from build123d import *

# Parameters (mm, degrees)
SKETCH3_R           = 2.032
SKETCH3_W           = 0.76159928
SKETCH3_H           = 0.76159928
SKETCH3_W_2         = 1.204804675
SKETCH3_H_2         = 2.605195325
SKETCH3_W_3         = 2.605195325
SKETCH3_H_3         = 1.204804675
BOSS_EXTRUDE3_DEPTH = 914.4


with BuildPart() as part:
    # Sketch3 → Boss-Extrude3 (new body)
    with BuildSketch(Plane.XY):
        with BuildLine():
            ThreePointArc((9.717596045, 8.176694142), (8.980256121, 8.980256121), (8.176694142, 9.717596045))
            Line((8.176694142, 9.717596045), (4.57240072, 9.717596045))
            Line((4.57240072, 9.717596045), (4.57240072, 7.11240072))
            Line((4.57240072, 7.11240072), (4.57240072, 5.334))
            Line((4.57240072, 5.334), (5.334, 5.334))
            Line((5.334, 5.334), (5.334, 4.57240072))
            Line((5.334, 4.57240072), (7.11240072, 4.57240072))
            Line((7.11240072, 4.57240072), (9.717596045, 4.57240072))
            Line((9.717596045, 4.57240072), (9.717596045, 8.176694142))
        make_face()
        with Locations((6.914797213, 6.914797213)):
            Circle(SKETCH3_R, mode=Mode.SUBTRACT)
        with Locations((4.95320036, 4.95320036)):
            Rectangle(SKETCH3_W, SKETCH3_H)
        Polygon((4.57240072, 5.334), (3.367596045, 5.334), (3.367596045, 4.191), (4.191, 4.191), (4.191, 3.367596045), (5.334, 3.367596045), (5.334, 4.57240072), (4.57240072, 4.57240072), align=None)
        with BuildLine():
            Line((3.367596045, 5.334), (-3.367596045, 5.334))
            Line((-3.367596045, 5.334), (-3.367596045, 4.191))
            Line((-3.367596045, 4.191), (-2.262062168, 4.191))
            ThreePointArc((-2.262062168, 4.191), (0, 4.7625), (2.262062168, 4.191))
            Line((2.262062168, 4.191), (3.367596045, 4.191))
            Line((3.367596045, 4.191), (3.367596045, 5.334))
        make_face()
        with BuildLine():
            Line((5.334, 3.367596045), (4.191, 3.367596045))
            Line((4.191, 3.367596045), (4.191, 2.262062168))
            ThreePointArc((4.191, 2.262062168), (4.617415064, 1.16656949), (4.7625, 0))
            ThreePointArc((4.7625, 0), (4.617415064, -1.16656949), (4.191, -2.262062168))
            Line((4.191, -2.262062168), (4.191, -3.367596045))
            Line((4.191, -3.367596045), (5.334, -3.367596045))
            Line((5.334, -3.367596045), (5.334, 3.367596045))
        make_face()
        with Locations((3.969998383, 8.414998383)):
            Rectangle(SKETCH3_W_2, SKETCH3_H_2)
        with Locations((8.414998383, 3.969998383)):
            Rectangle(SKETCH3_W_3, SKETCH3_H_3)
        with BuildLine():
            Line((4.57240072, -9.717596045), (8.176694142, -9.717596045))
            ThreePointArc((8.176694142, -9.717596045), (8.980256121, -8.980256121), (9.717596045, -8.176694142))
            Line((9.717596045, -8.176694142), (9.717596045, -4.57240072))
            Line((9.717596045, -4.57240072), (7.11240072, -4.57240072))
            Line((7.11240072, -4.57240072), (5.334, -4.57240072))
            Line((5.334, -4.57240072), (5.334, -5.334))
            Line((5.334, -5.334), (4.57240072, -5.334))
            Line((4.57240072, -5.334), (4.57240072, -7.11240072))
            Line((4.57240072, -7.11240072), (4.57240072, -9.717596045))
        make_face()
        with Locations((6.914797213, -6.914797213)):
            Circle(SKETCH3_R, mode=Mode.SUBTRACT)
        with Locations((4.95320036, -4.95320036)):
            Rectangle(SKETCH3_W, SKETCH3_H)
        with Locations((8.414998383, -3.969998383)):
            Rectangle(SKETCH3_W_3, SKETCH3_H_3)
        with Locations((3.969998383, -8.414998383)):
            Rectangle(SKETCH3_W_2, SKETCH3_H_2)
        Polygon((3.367596045, -4.191), (3.367596045, -5.334), (4.57240072, -5.334), (4.57240072, -4.57240072), (5.334, -4.57240072), (5.334, -3.367596045), (4.191, -3.367596045), (4.191, -4.191), align=None)
        with BuildLine():
            Line((-2.262062168, -4.191), (-3.367596045, -4.191))
            Line((-3.367596045, -4.191), (-3.367596045, -5.334))
            Line((-3.367596045, -5.334), (3.367596045, -5.334))
            Line((3.367596045, -5.334), (3.367596045, -4.191))
            Line((3.367596045, -4.191), (2.262062168, -4.191))
            ThreePointArc((2.262062168, -4.191), (0, -4.7625), (-2.262062168, -4.191))
        make_face()
        with Locations((-4.95320036, -4.95320036)):
            Rectangle(SKETCH3_W, SKETCH3_H)
        Polygon((-4.191, -3.367596045), (-5.334, -3.367596045), (-5.334, -4.57240072), (-4.57240072, -4.57240072), (-4.57240072, -5.334), (-3.367596045, -5.334), (-3.367596045, -4.191), (-4.191, -4.191), align=None)
        with BuildLine():
            Line((-5.334, -4.57240072), (-7.11240072, -4.57240072))
            Line((-7.11240072, -4.57240072), (-9.717596045, -4.57240072))
            Line((-9.717596045, -4.57240072), (-9.717596045, -8.176694142))
            ThreePointArc((-9.717596045, -8.176694142), (-8.980256121, -8.980256121), (-8.176694142, -9.717596045))
            Line((-8.176694142, -9.717596045), (-4.57240072, -9.717596045))
            Line((-4.57240072, -9.717596045), (-4.57240072, -7.11240072))
            Line((-4.57240072, -7.11240072), (-4.57240072, -5.334))
            Line((-4.57240072, -5.334), (-5.334, -5.334))
            Line((-5.334, -5.334), (-5.334, -4.57240072))
        make_face()
        with Locations((-6.914797213, -6.914797213)):
            Circle(SKETCH3_R, mode=Mode.SUBTRACT)
        with Locations((-3.969998383, -8.414998383)):
            Rectangle(SKETCH3_W_2, SKETCH3_H_2)
        with Locations((-8.414998383, -3.969998383)):
            Rectangle(SKETCH3_W_3, SKETCH3_H_3)
        with BuildLine():
            Line((-4.191, 3.367596045), (-5.334, 3.367596045))
            Line((-5.334, 3.367596045), (-5.334, -3.367596045))
            Line((-5.334, -3.367596045), (-4.191, -3.367596045))
            Line((-4.191, -3.367596045), (-4.191, -2.262062168))
            ThreePointArc((-4.191, -2.262062168), (-4.7625, 0), (-4.191, 2.262062168))
            Line((-4.191, 2.262062168), (-4.191, 3.367596045))
        make_face()
        with Locations((-4.95320036, 4.95320036)):
            Rectangle(SKETCH3_W, SKETCH3_H)
        Polygon((-4.57240072, 4.57240072), (-5.334, 4.57240072), (-5.334, 3.367596045), (-4.191, 3.367596045), (-4.191, 4.191), (-3.367596045, 4.191), (-3.367596045, 5.334), (-4.57240072, 5.334), align=None)
        with BuildLine():
            Line((-9.717596045, 4.57240072), (-7.11240072, 4.57240072))
            Line((-7.11240072, 4.57240072), (-5.334, 4.57240072))
            Line((-5.334, 4.57240072), (-5.334, 5.334))
            Line((-5.334, 5.334), (-4.57240072, 5.334))
            Line((-4.57240072, 5.334), (-4.57240072, 7.11240072))
            Line((-4.57240072, 7.11240072), (-4.57240072, 9.717596045))
            Line((-4.57240072, 9.717596045), (-8.176694142, 9.717596045))
            ThreePointArc((-8.176694142, 9.717596045), (-8.980256121, 8.980256121), (-9.717596045, 8.176694142))
            Line((-9.717596045, 8.176694142), (-9.717596045, 4.57240072))
        make_face()
        with Locations((-6.914797213, 6.914797213)):
            Circle(SKETCH3_R, mode=Mode.SUBTRACT)
        with Locations((-3.969998383, 8.414998383)):
            Rectangle(SKETCH3_W_2, SKETCH3_H_2)
        with Locations((-8.414998383, 3.969998383)):
            Rectangle(SKETCH3_W_3, SKETCH3_H_3)
    extrude(amount=BOSS_EXTRUDE3_DEPTH)


solid = part.part
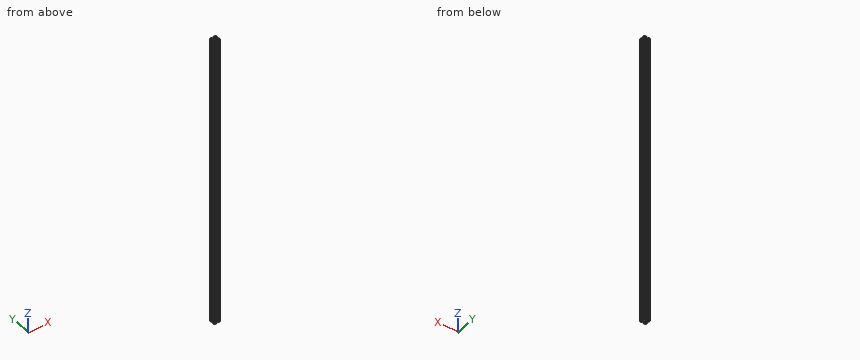
Work out the finished part from the listing and answer in its coordinate system (mm). Give positions to 0.01 mm unless a question says otherwise; leave off trailing zeros. Use a Markdown table: item, result. Add a question column.
1) The part is cut by section A-A, the plane z = 788. Count the separate pieces of the cut face and the enclosed holes in it, plus the area to 3 significant figures.
2) Consider line 1 along X through (y, z) = (6.5, 138.5); line 2 along Y through (x, z) = (3.5, 511); line 3 along X through (y, z) = (7.75, 384). Determine where each line is inside the solid, lowest interval first.
3) Each of these flat-tipped pins is pushed along its axis until it touches: P1, Ø3.5, axis at x = -6.91, y = -6.91, coming from the +Z side; P2, Ø0.8, axis at x = -9, z = 324, coming from the +Y side; P3, Ø0.8, axis at y = -9, z = 264.5, coming from the -X side. Where does it stop, or does it pass through?
Reported:
| question | item | result |
|---|---|---|
| 1 | separate pieces | 1 |
| 1 | enclosed holes | 5 |
| 1 | area | 109 mm^2 |
| 2 | line 1 | x = -9.72 to -8.9, -4.93 to -4.57, 4.57 to 4.93, 8.9 to 9.72 |
| 2 | line 2 | y = -9.72 to -7.11, -5.33 to -4.19, 4.19 to 5.33, 7.11 to 9.72 |
| 2 | line 3 | x = -9.72 to -8.77, -5.06 to -3.37, 3.37 to 5.06, 8.77 to 9.72 |
| 3 | P1 | passes through |
| 3 | P2 | stops at y = 9.35 |
| 3 | P3 | stops at x = -9.35 |
